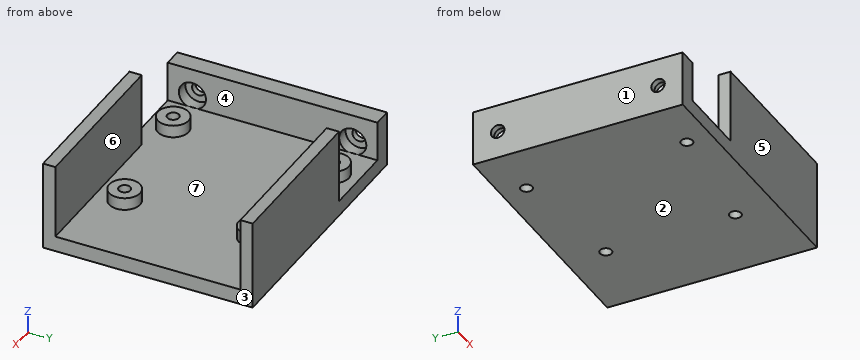
from build123d import *

# Parameters (mm, degrees)
SKETCH1_W                     = 42
SKETCH1_H                     = 34
BOSS_EXTRUDE1_DEPTH           = 2.5
BOSS_EXTRUDE2_DEPTH           = 12
SKETCH3_W                     = 12
SKETCH3_H                     = 34
CUT_EXTRUDE1_DEPTH            = 12
CBORE_FOR_M2_SHCS1_AT_2_COUNT = 2
CBORE_FOR_M2_SHCS1_AT_2_PITCH = 26
SKETCH8_W                     = 3
SKETCH8_H                     = 34
CUT_EXTRUDE2_DEPTH            = 5.5
SKETCH9_R                     = 2.5
BOSS_EXTRUDE3_DEPTH           = 2
SKETCH10_R                    = 0.95
CUT_EXTRUDE3_DEPTH            = 4.5


with BuildPart() as part:
    # Sketch1 → Boss-Extrude1 (new body)
    with BuildSketch(Plane.XY):
        with Locations((21, 17)):
            Rectangle(SKETCH1_W, SKETCH1_H)
    extrude(amount=BOSS_EXTRUDE1_DEPTH)

    # Sketch2 → Boss-Extrude2 (add)
    with BuildSketch(Plane.XY.offset(2.5)):
        Polygon((0, 34), (42, 34), (42, 32), (3, 32), (3, 2), (42, 2), (42, 0), (0, 0), align=None)
    extrude(amount=BOSS_EXTRUDE2_DEPTH)

    # Sketch3 → Cut-Extrude1 (cut)
    with BuildSketch(Plane.XY.offset(14.5)):
        with Locations((9, 17)):
            Rectangle(SKETCH3_W, SKETCH3_H)
    extrude(amount=-CUT_EXTRUDE1_DEPTH, mode=Mode.SUBTRACT)

    # Sketch5 → CBORE for M2 SHCS1 (revolve, cut)
    with BuildSketch(Plane(origin=(3, 4, 4.5), x_dir=(0, 0, -1), z_dir=(0, 1, 0))):
        Polygon((0, 0), (0, 3), (1.1, 3), (1.1, 2), (2.2, 2), (2.2, 0), align=None)
    cbore_for_m2_shcs1 = revolve(axis=Axis((9.35, 4, 4.5), (-1, 0, 0)), mode=Mode.SUBTRACT)

    # CBORE for M2 SHCS1 at 2: CBORE for M2 SHCS1 ×2
    with Locations(*[(0, i * CBORE_FOR_M2_SHCS1_AT_2_PITCH, 0) for i in range(1, CBORE_FOR_M2_SHCS1_AT_2_COUNT)]):
        add(cbore_for_m2_shcs1, mode=Mode.SUBTRACT)

    # Sketch8 → Cut-Extrude2 (cut)
    with BuildSketch(Plane.XY.offset(14.5)):
        with Locations((1.5, 17)):
            Rectangle(SKETCH8_W, SKETCH8_H)
    extrude(amount=-CUT_EXTRUDE2_DEPTH, mode=Mode.SUBTRACT)

    # Sketch9 → Boss-Extrude3 (add)
    with BuildSketch(Plane.XY.offset(2.5)):
        with Locations(Location((9, 30, 0), (0, 0, 180))):
            Circle(SKETCH9_R)
        with Locations(Location((9, 4, 0), (0, 0, 180))):
            Circle(SKETCH9_R)
        with Locations(Location((29, 27.5, 0), (0, 0, 180))):
            Circle(SKETCH9_R)
        with Locations(Location((29, 6.5, 0), (0, 0, 180))):
            Circle(SKETCH9_R)
    extrude(amount=BOSS_EXTRUDE3_DEPTH)

    # Sketch10 → Cut-Extrude3 (cut)
    with BuildSketch(Plane.XY.offset(4.5)):
        with Locations((9, 30)):
            Circle(SKETCH10_R)
        with Locations((9, 4)):
            Circle(SKETCH10_R)
        with Locations((29, 27.5)):
            Circle(SKETCH10_R)
        with Locations((29, 6.5)):
            Circle(SKETCH10_R)
    extrude(amount=-CUT_EXTRUDE3_DEPTH, mode=Mode.SUBTRACT)


solid = part.part
CAD build for the part. Positions are in the model's coordinates, mm. Face numbers are marked on the shaded views. A direction names the side the tool comes from. Give positions to 0.01 mm unless a question says otherwise; leave off trailing zeros. Order: outer loops, then holes, each group sorted by start corner. A loop starts at its lowest first (then second) coordinate and runs counter-clockwise, first axis right, second up. Notation, with made-up numbers: (3, 86) - (38, 86) arc R10 ccw to (38, 102) - close; hole circle Ø8 at (83.5, 42.5). An arc over 180 degrees is marked (long way). Write each question's results on one line, items separated by ' | '.
1. Saw through at B-B on z = 7.5. List the corners of the cut face in (x, y), and give its area (3 significant figures).
Calculated:
outline: (0, 0) - (3, 0) - (3, 34) - (0, 34) - close; (15, 0) - (42, 0) - (42, 2) - (15, 2) - close; (15, 32) - (42, 32) - (42, 34) - (15, 34) - close | area: 210 mm2
2. Probe L1, parallel to Y at x = 1.6, z = 4.5; L2, parallel to Y at x = 29, z = 3.2; L3, parallel to Y at x = 0.35, z = 4.5. List the from-to ranges inside material, lowest first. Write a range as from..to.
Calculated:
L1: y = 0..1.8, 6.2..27.8, 32.2..34 | L2: y = 0..2, 4..5.55, 7.45..9, 25..26.55, 28.45..30, 32..34 | L3: y = 0..2.9, 5.1..28.9, 31.1..34
3. Saw through at C-C on x = 9. List the corners of the cut face in (y, z), and give its area (3 significant figures).
Calculated:
outline: (0, 0) - (3.05, 0) - (3.05, 4.5) - (1.5, 4.5) - (1.5, 2.5) - (0, 2.5) - close; (4.95, 0) - (29.05, 0) - (29.05, 4.5) - (27.5, 4.5) - (27.5, 2.5) - (6.5, 2.5) - (6.5, 4.5) - (4.95, 4.5) - close; (30.95, 0) - (34, 0) - (34, 2.5) - (32.5, 2.5) - (32.5, 4.5) - (30.95, 4.5) - close | area: 87.9 mm2
4. Saw through at D-D on y = 12.5. List the corners of the cut face in (x, z), and give its area (4 significant figures).
Calculated:
outline: (0, 0) - (42, 0) - (42, 2.5) - (3, 2.5) - (3, 9) - (0, 9) - close | area: 124.5 mm2
5. 3-axis set-ups, long thin cutter, end or side, ignore diameter. For the marked faces 5, 6 and 7: which of +Z, -Z, +X, -X, +Y, -Y reach the whole face in a straight line?
Calculated:
face 5: +Z, -Z, +X, -X, -Y | face 6: +Z, +X | face 7: +Z
6. Pull direction X, two halves, no side cores. Call the marked faces 1, 2, 3 and 4: released by +X, released by -X, zero draft, split by the parting line, or undercut.
Calculated:
face 1: released by -X | face 2: zero draft | face 3: released by +X | face 4: undercut
7. Pin check, flat tips, straight feed: pin 1 (2 mm diameter, centred on x = 9, y = 30, fed in from +Z); pin 2 (3 mm diameter, centred on x = 21.5, y = 22, fed in from +Z); pin 3 (3 mm diameter, centred on x = 33, y = 28, fed in from -Z); pin 4 (3.5 mm diameter, centred on x = 1, y = 11.5, fed in from +Z). Stop position of each tip, or through.
Calculated:
pin 1: stops at z = 4.5 | pin 2: stops at z = 2.5 | pin 3: stops at z = 0 | pin 4: stops at z = 9
8. Saw through at A-A on x = 29. List the corners of the cut face in (y, z), and give its area (3 significant figures).
Calculated:
outline: (0, 0) - (5.55, 0) - (5.55, 4.5) - (4, 4.5) - (4, 2.5) - (2, 2.5) - (2, 14.5) - (0, 14.5) - close; (7.45, 0) - (26.55, 0) - (26.55, 4.5) - (25, 4.5) - (25, 2.5) - (9, 2.5) - (9, 4.5) - (7.45, 4.5) - close; (28.45, 0) - (34, 0) - (34, 14.5) - (32, 14.5) - (32, 2.5) - (30, 2.5) - (30, 4.5) - (28.45, 4.5) - close | area: 136 mm2
